Geometry check sheet. Reference: the model listing, model coordinates, mm. A direction names the side the tool comes from. Give positions to 0.01 mm unless a question says otherwise; leave off trailing zeros. Order: outer loops, then holes, each group sorted by start corner. A loop starts at its lowest first (then second) coordinate and runs counter-clockwise, first axis right, second up. Notation, with made-up numbers: M -1,82 L 38,82 A26 ccw 38,121 Z; hole C -15.5,54 d11. An arc over 180 degrees is marked long. Answer as CSV lines item,"result". Start each with the question number.
Q1. Mould release check, pull along Y, two halves, no side actions. Record for faces 4 (the flat face through (16, 8, 0)), 5 (the flat face through (0, 32.996, 25)), 6 (the flat face through (28.44, -16.73, 25.04)), 7 (the flat face through (9.77, -13.16, 12.52)): +Y half, -Y half, draft (parallel to the pull), parting line (faces both ways), or undercut.
Q2. Section check B-B, the plane y = 12. Record the boundary of the cut face in (x, z).
Q3. Section check A-A, the plane z = 32. Record the boundary of the cut face in (x, y), then the cut area to 3 significant figures.
Q4. Section check D-D, the plane y = -23.5. Record the boundary of the cut face in (x, z), then the cut area to 3 significant figures.
Q5. Thickness scan on line 1 (Y direction, x = 0, z = 44.25); line 2 (X direction, y = -11, z = 39.5); line 3 (Y direction, x = 8.5, z = 30). Record the ranges inside material, lowest first.
Q6. Section check C-C, the plane x = 4. Record the boundary of the cut face in (y, z), then the cut area to 3 significant figures.
Q7. Go/stop test with flat-tipped pins: pin 1 (5 mm diameter, centred on x = -24.5, z = 30.5, fed in from -Y); pin 2 (2 mm diameter, centred on y = 24.5, z = 38, fed in from +X); pin 3 (10 mm diameter, centred on x = -29, z = 22.5, fed in from +Y). Record where each tip stops, or that it passes through.
Q8. Set-up check for faces 1 (the flat face through (0, 16.388, 13)), 2 (the flat face through (16.8, -19.4, 50.8)), 3 (the flat face through (5, -17, 25.4)): record each of +Z, -Z, +X, -X, +Y, -Y from which the full face is reachable in a straight line by a thin tool's end or side.
```python
from build123d import *

# Parameters (mm, degrees)
F1_DEPTH = 25.4
F3_DEPTH = 25.4
F4_R     = 25.4
F5_DEPTH = 25.4


with BuildPart() as f1:
    # F0 (on Top) → F1 (new body)
    with BuildSketch(Plane.XY):
        Polygon((19.05, 32.995568), (-19.05, 32.995568), (-38.1, 0), (-19.05, -32.995568), (19.05, -32.995568), (38.1, 0), align=None)
        Polygon((-19.264717, -6.259486), (-11.90625, 16.387547), (11.90625, 16.387547), (19.264717, -6.259486), (0, -20.256122), align=None, mode=Mode.SUBTRACT)
    extrude(amount=F1_DEPTH)

    # F2 (on face) → F3 (join)
    with BuildSketch(Plane.XY.offset(25.4)):
        Polygon((0, -20.256122), (19.264717, -6.259486), (11.90625, 16.387547), (-11.90625, 16.387547), (-19.264717, -6.259486), align=None)
        Polygon((19.05, -32.995568), (38.1, 0), (19.05, 32.995568), (-19.05, 32.995568), (-38.1, 0), (-19.05, -32.995568), align=None)
        Polygon((11.90625, 16.387547), (19.264717, -6.259486), (0, -20.256122), (-19.264717, -6.259486), (-11.90625, 16.387547), align=None, mode=Mode.SUBTRACT)
    extrude(amount=F3_DEPTH)

    # F4 (on face) → F5 (cut)
    with BuildSketch(Plane.XY.offset(50.8)):
        Circle(F4_R)
    extrude(amount=-F5_DEPTH, mode=Mode.SUBTRACT)


solid = f1.part
```
Answer block:
1,face 4,"draft"
1,face 5,"+Y half"
1,face 6,"-Y half"
1,face 7,"undercut"
2,outline,"M -31.17,0 L -13.33,0 L -13.33,25.4 L -22.39,25.4 L -22.39,50.8 L -31.17,50.8 Z; M 13.33,0 L 31.17,0 L 31.17,50.8 L 22.39,50.8 L 22.39,25.4 L 13.33,25.4 Z"
3,outline,"M -38.1,0 L -19.05,-33 L 19.05,-33 L 38.1,0 L 19.05,33 L -19.05,33 Z; hole C 0,0 d50.8"
3,area,"1,740 mm2"
4,outline,"M -24.53,0 L 24.53,0 L 24.53,50.8 L 9.64,50.8 L 9.64,25.4 L -9.64,25.4 L -9.64,50.8 L -24.53,50.8 Z"
4,area,"2,000 mm2"
5,line 1,"y = -33 to -25.4, 25.4 to 33"
5,line 2,"x = -31.75 to -22.89, 22.89 to 31.75"
5,line 3,"y = -33 to -23.94, 23.94 to 33"
6,outline,"M -33,0 L -17.35,0 L -17.35,25.4 L -25.08,25.4 L -25.08,50.8 L -33,50.8 Z; M 16.39,0 L 33,0 L 33,50.8 L 25.08,50.8 L 25.08,25.4 L 16.39,25.4 Z"
6,area,"1,220 mm2"
7,pin 1,"stops at y = -27.89"
7,pin 2,"stops at x = 24.53"
7,pin 3,"stops at y = 24.42"
8,face 1,"+Z, -Z"
8,face 2,"+Z, +X, -X, +Y, -Y"
8,face 3,"+Z"
